Autodesk Inventor part; units mm, degrees
ref_plane "YZ Plane" through (0, 0, 0) normal (1, 0, 0) x (0, 1, 0)
ref_plane "XZ Plane" through (0, 0, 0) normal (0, 1, 0) x (-1, 0, 0)
ref_plane "XY Plane" through (0, 0, 0) normal (0, 0, 1) x (1, 0, 0)
sketch "スケッチ1" plane through (0, 0, 0) normal (0, 0, 1) x (1, 0, 0)
  line L0 (18.4549, -8.1589) -> (14.4552, -8.1589)
  arc A0 (18.4549, -8.1589) -> (20.0703, -6.5435) centre (18.4549, -6.5435) ccw
  line L1 (20.0703, -2.0624) -> (20.0703, -6.5435)
  line L2 (18.0495, -0.0417) -> (-1.0589, -0.0417)
  arc A1 (-1.0589, -0.0417) -> (-2.9016, -1.8843) centre (-1.0589, -1.8843) ccw
  line L3 (-2.9016, -1.8843) -> (-2.9016, -6.5559)
  arc A2 (-2.9016, -6.5559) -> (-0.7003, -8.7571) centre (-0.7003, -6.5559) ccw
  arc A3 (26.8987, -33.0319) -> (28.4367, -33.0608) centre (27.7277, -29.8571) ccw
  line L4 (30.1493, -31.6136) -> (28.4367, -33.0608)
  arc A4 (30.1493, -31.6136) -> (31.6494, -28.7162) centre (32.5816, -31.0359) ccw
  line L5 (31.6494, -28.7162) -> (14.4552, -8.1589)
  circle A5 centre (16.1123, -4.0657) radius 2.5
  line L6 (7.6373, -0.9827) -> (1.1644, -0.9827)
  arc A6 (7.6373, -7.2327) -> (7.6373, -0.9827) centre (7.6373, -4.1077) ccw
  arc A7 (1.1644, -0.9827) -> (1.1644, -7.2327) centre (1.1644, -4.1077) ccw
  line L7 (26.8987, -33.0319) -> (6.5951, -8.7571)
  line L8 (-0.7003, -8.7571) -> (6.5951, -8.7571)
  arc A8 (20.0703, -2.0624) -> (18.0495, -0.0417) centre (18.0495, -2.0624) ccw
  line L9 (1.1644, -7.2327) -> (7.6373, -7.2327)
  line L10 (13.6123, -4.0657) -> (13.6123, 1.3375)
  line L11 (10.7623, -4.0657) -> (10.7623, 0.9924)
  point P0 (0, 0)
  point P1 (0, 0)
  dimension "d0" = 5
  dimension "d1" = 3.125
  dimension "d2" = 4.8539
  dimension "d3" = 4.066
  dimension "d4" = 4.066
  dimension "d5" = 90
  dimension "d6" = 90
  dimension "d7" = 3.125
  dimension "d8" = 3.9579
  dimension "d9" = 22.9718
  dimension "d10" = 2.5
  dimension "d11" = 2.85
extrude "押し出し1" add sketch "スケッチ1" along normal blind 10
sketch "スケッチ2" plane through (0, 0, 0) normal (0, 0, -1) x (-1, 0, 0)
  arc A0 (-7.6373, -0.9827) -> (-7.6373, -7.2327) centre (-7.6373, -4.1077) ccw
  line L0 (-7.6373, -0.9827) -> (-1.1644, -0.9827)
  arc A1 (-1.1644, -7.2327) -> (-1.1644, -0.9827) centre (-1.1644, -4.1077) ccw
  line L1 (-1.1644, -7.2327) -> (-7.6373, -7.2327)
  circle A2 centre (-16.1123, -4.0657) radius 2.5
  line L2 (-14.4552, -8.1589) -> (-18.4549, -8.1589)
  line L3 (-31.6494, -28.7162) -> (-14.4552, -8.1589)
  arc A3 (-31.6494, -28.7162) -> (-30.1493, -31.6136) centre (-32.5816, -31.0359) ccw
  line L4 (-28.4367, -33.0608) -> (-30.1493, -31.6136)
  arc A4 (-28.4367, -33.0608) -> (-26.8987, -33.0319) centre (-27.7277, -29.8571) ccw
  line L5 (-6.5951, -8.7571) -> (-26.8987, -33.0319)
  line L6 (0.7003, -8.7571) -> (-6.5951, -8.7571)
  arc A5 (0.7003, -8.7571) -> (2.9016, -6.5559) centre (0.7003, -6.5559) ccw
  line L7 (2.9016, -1.8843) -> (2.9016, -6.5559)
  arc A6 (2.9016, -1.8843) -> (1.0589, -0.0417) centre (1.0589, -1.8843) ccw
  line L8 (-18.0495, -0.0417) -> (1.0589, -0.0417)
  arc A7 (-18.0495, -0.0417) -> (-20.0703, -2.0624) centre (-18.0495, -2.0624) ccw
  line L9 (-20.0703, -6.5435) -> (-20.0703, -2.0624)
  arc A8 (-20.0703, -6.5435) -> (-18.4549, -8.1589) centre (-18.4549, -6.5435) ccw
  circle A9 centre (-32.5816, -31.0359) radius 2.5
  point P0 (0, 0)
extrude "押し出し2" add sketch "スケッチ2" along normal blind 10 contours A9 A3
sketch "スケッチ3" plane through (0, 0, 10) normal (0, 0, 1) x (1, 0, 0)
  arc A0 (7.6373, -7.2327) -> (7.6373, -0.9827) centre (7.6373, -4.1077) ccw
  circle A1 centre (16.1123, -4.0657) radius 2.5
  line L0 (18.0495, -0.0417) -> (-1.0589, -0.0417)
  line L1 (14.2688, -7.695) -> (18.4549, -7.695)
  line L2 (7.8873, -8.8011) -> (13.8903, -8.8011)
  line L3 (13.8903, -8.8011) -> (29.8014, -27.8243)
  line L4 (29.8014, -27.8243) -> (26.6112, -31.1873)
  line L5 (26.6112, -31.1873) -> (7.8873, -8.8011)
  line L6 (7.8873, -8.8011) -> (13.8903, -8.8011)
  arc A2 (7.6373, -7.2327) -> (7.6373, -0.9827) centre (7.6373, -4.1077) ccw
  line L7 (7.6373, -7.2327) -> (1.1644, -7.2327)
  arc A3 (1.1644, -0.9827) -> (1.1644, -7.2327) centre (1.1644, -4.1077) ccw
  line L8 (1.1644, -0.9827) -> (7.6373, -0.9827)
  circle A4 centre (16.1123, -4.0657) radius 2.5
  line L9 (14.2688, -7.695) -> (18.4549, -7.695)
  arc A5 (18.4549, -7.695) -> (20.0703, -6.0796) centre (18.4549, -6.0796) ccw
  line L10 (20.0703, -6.0796) -> (20.0703, -2.0624)
  arc A6 (20.0703, -2.0624) -> (18.0495, -0.0417) centre (18.0495, -2.0624) ccw
  line L11 (18.0495, -0.0417) -> (-1.0589, -0.0417)
  arc A7 (-1.0589, -0.0417) -> (-2.9016, -1.8843) centre (-1.0589, -1.8843) ccw
  line L12 (-2.9016, -1.8843) -> (-2.9016, -6.5999)
  arc A8 (-2.9016, -6.5999) -> (-0.7003, -8.8011) centre (-0.7003, -6.5999) ccw
  line L13 (-0.7003, -8.8011) -> (6.5837, -8.8011)
  line L14 (6.5837, -8.8011) -> (26.8872, -33.0759)
  arc A9 (26.8872, -33.0759) -> (27.9503, -33.1763) centre (27.7277, -29.8571) ccw
  line L15 (27.9503, -33.1763) -> (29.6628, -31.7291)
  arc A10 (29.6628, -31.7291) -> (31.463, -28.2522) centre (32.5816, -31.0359) ccw
  line L16 (31.463, -28.2522) -> (14.2688, -7.695)
  arc A11 (9.5454, -7.2327) -> (9.5355, -0.9767) centre (7.6373, -4.1077) ccw
  arc A12 (14.3143, -0.9767) -> (14.4552, -7.2327) centre (16.1123, -4.0657) ccw
  line L17 (9.5454, -7.2327) -> (14.4552, -7.2327)
  line L18 (9.5355, -0.9767) -> (14.3143, -0.9767)
  point P0 (0, 0)
  point P1 (0, 0)
extrude "押し出し3" cut sketch "スケッチ3" against normal blind 1 contours A11 L18 A12 L17
sketch "スケッチ4" plane through (0, 0, 10) normal (0, 0, 1) x (1, 0, 0)
  line L0 (6.5837, -8.8011) -> (26.8872, -33.0759)
  line L1 (31.463, -28.2522) -> (14.2688, -7.695)
  line L2 (6.5837, -8.8011) -> (15.194, -8.8011)
  line L3 (26.8872, -33.0759) -> (31.463, -28.2522)
  line L4 (31.463, -28.2522) -> (15.194, -8.8011)
  line L5 (26.8872, -33.0759) -> (6.5837, -8.8011)
  line L6 (25.9184, -31.9176) -> (30.4942, -27.0939)
  line L7 (26.6112, -31.1873) -> (7.8873, -8.8011)
  line L8 (29.8014, -27.8243) -> (13.8903, -8.8011)
  point P0 (0, 0)
  point P1 (0, 0)
  dimension "d18" = 1.5
  dimension "d19" = 1
  dimension "d20" = 1
extrude "押し出し4" cut sketch "スケッチ4" against normal blind 1 contours L2 L8 L6 L7
sketch "スケッチ5" plane through (0, 0, 10) normal (0, 0, 1) x (1, 0, 0)
  arc A0 (30.1493, -31.6136) -> (31.6494, -28.7162) centre (32.5816, -31.0359) ccw
  circle A1 centre (32.5816, -31.0359) radius 1.5
  point P0 (0, 0)
  point P1 (0, 0)
  dimension "d26" = 1
extrude "押し出し5" cut sketch "スケッチ5" against normal blind 1
equation "\"d4\" = d3"
equation "\"d7\" = d1"
properties part number "finger_4_5mm"
Input: part model. Units: mm. Frame: model coordinates. A direction names the side the tool comes from. Coordinates: 2 decimals unless noted, no trailing zeros. Loops run counter-clockwise (first coordinate to the right, second up) from the corner with the lowest first, then second, coordinate; pieces in that order, holes last. Notation, with made-up numbers: M 77,-7.75 L 128,-7.75 A15 ccw 128,1.25 Z; hole C 85,4 d11. An arc over 180 degrees is marked long. Use a Markdown table: item, result. Add a question column.
1) Section B-B, the plane y = -17. Return the cut outline in (x, z), plus the area to 3 significant figures.
2) Section D-D, the plane x = 22. Return the cut outline in (y, z).
3) Set-up query: faces 1 (the cylindrical face through (-1.96, -4.18, 4.93)), 2 (the flat face through (10.8, -8.801, 9.5)), 3 (the flat face through (9, -0.042, 5)), 4 (the cylindrical face through (-2.38, -0.6, 4.93)), 5 (the cylindrical face through (19.61, -7.67, 4.93)). Return all of +Z, -Z, +X, -X, +Y, -Y with unobstructed straight access to the full face (end or side cutting, diameter ignored); none if empty.
4) Draft query along Y for faces 6 (the cylindrical face through (19.463, -0.618, 4.93)), 7 (the flat face through (-2.902, -4, 5)), 8 (the flat face through (28.184, -29.529, 9.507)). Return one class per face: +Y half, -Y half, draft (parallel to the pull), parting line (faces both ways), or undercut.
5) Section C-C, the plane z = 8.5. Give the number of separate pieces and of enclosed holes in the cut face, plus the area to 3 significant figures.
6) Line query: L1, parallel to Y at x = 2, z = 6; L2, parallel to Z at x = 29.5, y = -30.5; L3, parallel to Z at x = 8.5, y = -9. Output: solid intervals per line, ascending. Write a range as from..to.
7) Pin query (flat end, axial travel): P1, Ø0.9, axis at x = 33, y = -31.5, coming from the +Z side; P2, Ø2, axis at x = 18, z = -1.5, coming from the -Y side; P3, Ø1.5, axis at x = 26.5, z = 5, coming from the +Y side; P4, Ø1.3, axis at y = -4, z = 7, coming from the +X side. Return the tip coordinate at first contact, or that it passes through.
8) Section A-A, the plane x = 5. Return the cut outline in (y, z), plus the area to 3 significant figures.
Answer below:
| question | item | result |
|---|---|---|
| 1 | outline | M 13.49,0 L 21.85,0 L 21.85,10 L 20.75,10 L 20.75,9 L 14.74,9 L 14.74,10 L 13.49,10 Z |
| 1 | area | 77.6 mm2 |
| 2 | outline | M -27.18,0 L -17.18,0 L -17.18,10 L -18.5,10 L -18.5,9 L -25.67,9 L -25.67,10 L -27.18,10 Z |
| 3 | face 1 | +Z, -Z |
| 3 | face 2 | +Z |
| 3 | face 3 | +Z, -Z, +X, -X, +Y |
| 3 | face 4 | +Z, -Z, -X, +Y |
| 3 | face 5 | +Z, -Z, +X |
| 4 | face 6 | +Y half |
| 4 | face 7 | draft |
| 4 | face 8 | undercut |
| 5 | separate pieces | 1 |
| 5 | enclosed holes | 2 |
| 5 | area | 311 mm2 |
| 6 | L1 | -8.76..-7.23, -0.98..-0.04 |
| 6 | L2 | 0..10 |
| 6 | L3 | 0..9 |
| 7 | P1 | z = 9 |
| 7 | P2 | through |
| 7 | P3 | y = -21.66 |
| 7 | P4 | x = 20.07 |
| 8 | outline | M -8.76,0 L -7.23,0 L -7.23,10 L -8.76,10 Z; M -0.98,0 L -0.04,0 L -0.04,10 L -0.98,10 Z |
| 8 | area | 24.7 mm2 |
